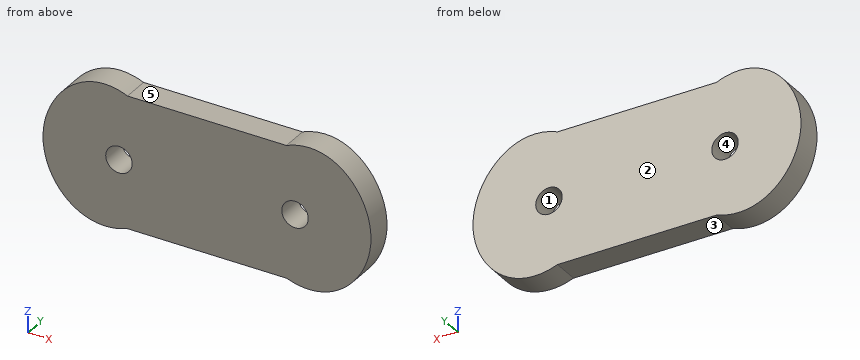
```python
from build123d import *

# Parameters (mm, degrees)
ESQUISSE2_R        = 1.5
BOSS_EXTRU_1_DEPTH = 3


with BuildPart() as part:
    # Esquisse2 → Boss.-Extru.1 (new body)
    with BuildSketch(Plane(origin=(0, 0, 0), x_dir=(1, 0, 0), z_dir=(0, 1, 0))):
        with BuildLine():
            Line((9, 7.5), (-9, 7.5))
            add(Edge.make_bspline(
                [(-9, 7.5), (-14.368679203, 9.540675776), (-22.864046294, 0.062993), (-14.222464977, -9.74400485), (-9, -7.5)],
                knots=[0, 0, 0, 0, 0.498997334, 1, 1, 1, 1], degree=3))
            Line((-9, -7.5), (9, -7.5))
            add(Edge.make_bspline(
                [(9, 7.5), (14.368679203, 9.540675776), (22.864046294, 0.062993), (14.222464977, -9.74400485), (9, -7.5)],
                knots=[0, 0, 0, 0, 0.498997334, 1, 1, 1, 1], degree=3))
        make_face()
        with Locations(Location((-9.973759583, 0, 0), (0, 0, 270))):
            Circle(ESQUISSE2_R, mode=Mode.SUBTRACT)
        with Locations(Location((9.973759583, 0, 0), (0, 0, 90))):
            Circle(ESQUISSE2_R, mode=Mode.SUBTRACT)
    extrude(amount=BOSS_EXTRU_1_DEPTH)


solid = part.part
```
Here's how the part is built. I have some questions about the finished solid (model axes, mm). Face numbers are marked on the shaded views. A direction names the side the tool comes from. Coordinates: 2 decimals unless noted, no trailing zeros. Order: outer loops, then holes, each group sorted by start corner. A loop starts at its lowest first (then second) coordinate and runs counter-clockwise, first axis right, second up.
1) Imagine slicing it at B-B on z = 0. State how many separate pieces and enclosed holes the cut face has, and give its area (3 significant figures).
2) Which directions (+Z, -Z, +X, -X, +Y, -Y) give clear straight access to the entire face, cutting with the end or side of a thin tool? Please do the marked faces 3, 4 and 5.
3) Imagine slicing it at A-A on x = -6. List the corners of the cut face in (y, z) for me.
4) We'd pull the mould along X, two halves only. Please class the marked faces 1 and 2: +X half, -X half, draft (parallel to the pull), parting line (faces both ways), or undercut.
5) Will these pins go through, and if not, where does the flat tip stop? pin 1 (1.5 mm diameter, centred on x = 2, y = 2, fed in from +Z); pin 2 (1.5 mm diameter, centred on x = 13.5, y = 2.5, fed in from -Z); pin 3 (2.5 mm diameter, centred on x = -9.97, z = 0, fed in from -Y); pin 4 (1 mm diameter, centred on x = 9, y = 0.5, fed in from -Z).
6) I need wall thicknesses on line 1 (X direction, y = 1.95, z = 0); line 2 (X direction, y = 2, z = -1); line 3 (Z direction, x = -5, y = 0.45). Which ranges of each line are inside material? Lowest first, please.
Response values:
1. separate pieces: 3
1. enclosed holes: 0
1. area: 93.5 mm2
2. face 3: -Z, +Y, -Y
2. face 4: +Y, -Y
2. face 5: +Z, +Y, -Y
3. outline: (0, -7.5) - (3, -7.5) - (3, 7.5) - (0, 7.5) - close
4. face 1: undercut
4. face 2: draft
5. pin 1: stops at z = 7.5
5. pin 2: stops at z = -7.87
5. pin 3: passes through
5. pin 4: stops at z = -7.67
6. line 1: x = -18.58 to -11.47, -8.47 to 8.47, 11.47 to 18.58
6. line 2: x = -18.52 to -11.09, -8.86 to 8.86, 11.09 to 18.52
6. line 3: z = -7.5 to 7.5
